```python
from build123d import *

# Parameters (mm, degrees)
F0_W            = 25
F0_H            = 50
F0_R            = 5
F1_DEPTH        = 15
F1_DEPTH_BACK   = 15
F2_COUNT        = 2
F2_ANGLE        = 90
F3_R            = 30
F4_DEPTH        = 50
F5_W            = 10
F5_H            = 64.0000030398
F6_DEPTH        = 50.0010001
F6_COPIES_COUNT = 4


# Not quite as in the source:
# - a pattern or mirror of a feature is missing from the dataset's text; its kind, count and spacing are read off the source's solid


with BuildPart() as f1:
    # F0 (on Front) → F1 (new body, two sides)
    with BuildSketch(Plane.XZ) as f1_sk:
        with Locations((-12.5, 25)):
            Rectangle(F0_W, F0_H)
        with Locations((12.5, 25)):
            Rectangle(F0_W, F0_H)
        with BuildLine():
            ThreePointArc((-25, 50), (-50, 25), (-25, 0))
            Line((-25, 0), (-25, 50))
        make_face()
        with Locations((-39.1249991953, 25)):
            Circle(F0_R, mode=Mode.SUBTRACT)
        with BuildLine():
            Line((25, 50), (25, 0))
            ThreePointArc((25, 0), (50, 25), (25, 50))
        make_face()
        with Locations((39.1249991953, 25)):
            Circle(F0_R, mode=Mode.SUBTRACT)
    extrude(amount=F1_DEPTH)
    extrude(f1_sk.sketch, amount=-F1_DEPTH_BACK)

    # F2: F1 ×2 about axis
    f2_axis = Axis((0, 0, 10.6249991804), (0, 0, 1))


with BuildPart() as f1_1:
    add(f1.part)
    for i in range(1, F2_COUNT):
        add(f1.part.rotate(f2_axis, i * F2_ANGLE / (F2_COUNT - 1)))

    # F3 (on face) → F4 (join, through all)
    with BuildSketch(Plane.XY.offset(50)):
        Circle(F3_R)
    extrude(amount=-F4_DEPTH)

    # F5 (on face) → F6 (cut, through all)
    with BuildSketch(Plane.XY.offset(50)):
        with Locations((0, 64.1250014305)):
            Rectangle(F5_W, F5_H)
    f6 = extrude(amount=-F6_DEPTH, mode=Mode.SUBTRACT)

    # F6_copies: F6 ×4 about axis
    f6_copies_axis = Axis((0, 0, 0), (0, 0, 1))
    for i in range(1, F6_COPIES_COUNT):
        add(f6.rotate(f6_copies_axis, i * 360 / F6_COPIES_COUNT), mode=Mode.SUBTRACT)


solid = f1_1.part
```
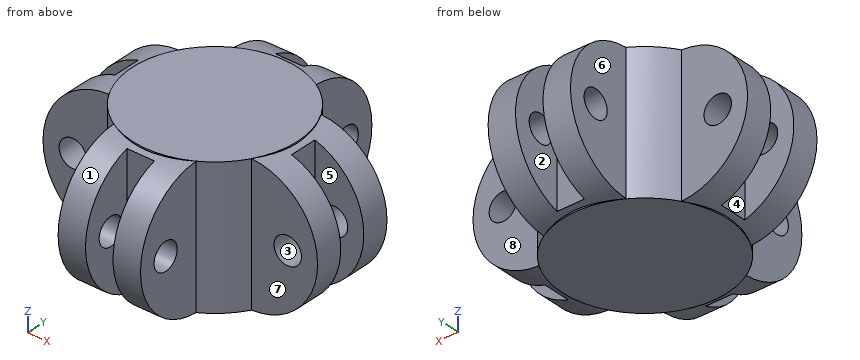
Design review of the part built by this model. Coordinates are the model's own, in mm. Face numbers are marked on the shaded views. A direction names the side the tool comes from. Round coordinates to 2 decimals unless told otherwise and drop trailing zeros. Write each loop counter-clockwise with the first axis right and the second up, starting at its lowest first coordinate (ties: lowest second). Pieces come first, ordered by that corner, then holes.
Item 1: We need section A-A on x = -13.5. Write out the cut boundary in (y, z) (3 decimals), and give its area (3 significant figures).
Item 2: We need section B-B on y = 35.5. Write out the cut boundary in (x, z), and give its area (3 significant figures).
Item 3: For the marked faces 4, 5, 6, 7 and 8, list the 3-axis set-ups (+Z, -Z, +X, -X, +Y, -Y) from which the entire face can be reached by the end or side of a thin tool; tool diameter is ignored.
Item 4: Clearance check with flat-ended pins moving along their axes: pin 1 Ø12 at (x, z) = (23.5, 41.5) entering from -Y; pin 2 Ø7 at (x, z) = (-40, 17) entering from +Y; pin 3 Ø3 at (y, z) = (-1, 28.5) entering from +X (3 decimals); pin 4 Ø6 at (x, z) = (-39.125, 25) entering from -Y. State where each tip first meets the part, or that it passes through.
Item 5: We need section D-D on y = -7. Write out the cut boundary in (x, z) (3 decimals).
Item 6: We need section C-C on z = 25. State how many separate pieces and enclosed holes the cut face has, and give its area (3 significant figures).
Item 7: The part is to be moulded in two halves that separate along Z. For the marked faces 1, 2 and 3, say which applies: +Z half, -Z half, draft (parallel to the pull), parting line (faces both ways), or undercut.
Item 8: For probe 1 along Y at (x, z) = (-12, 25) (3 decimals); probe 2 along X at (y, z) = (-34, 35); probe 3 along Y at (x, z) = (26.5, 28), list the stretches that pass through material, from the lowest coordinate up.
Returned:
1. outline: (-26.791, 0) - (26.791, 0) - (26.791, 0.064) arc R25 ccw to (26.791, 49.936) - (26.791, 50) - (-26.791, 50) - (-26.791, 49.936) arc R25 ccw to (-26.791, 0.064) - close; hole circle Ø10 at (-39.125, 25); hole circle Ø10 at (39.125, 25)
1. area: 4,310 mm2
2. outline: (-15, 2.31) - (-5, 2.31) - (-5, 21.56) - (-15, 21.56) - close; (-15, 28.44) - (-5, 28.44) - (-5, 47.69) - (-15, 47.69) - close; (5, 2.31) - (15, 2.31) - (15, 21.56) - (5, 21.56) - close; (5, 28.44) - (15, 28.44) - (15, 47.69) - (5, 47.69) - close
2. area: 770 mm2
3. face 4: +Z, -Z, -X
3. face 5: +Z, -Z, +X
3. face 6: +Z, -Z, -X, +Y
3. face 7: +Z, -Z, +X, -Y
3. face 8: +Z, -Z, +X, +Y
4. pin 1: stops at y = -24.37
4. pin 2: stops at y = 15
4. pin 3: stops at x = 32.125
4. pin 4: passes through
5. outline: (-29.172, 0) - (29.172, 0) - (29.172, 0.351) arc R25 ccw to (29.172, 49.649) - (29.172, 50) - (-29.172, 50) - (-29.172, 49.649) arc R25 ccw to (-29.172, 0.351) - close; hole circle Ø10 at (-39.125, 25); hole circle Ø10 at (39.125, 25)
6. separate pieces: 9
6. enclosed holes: 0
6. area: 3,870 mm2
7. face 1: parting line
7. face 2: draft
7. face 3: undercut
8. probe 1: y = -50 to -44.125, -34.125 to 34.125, 44.125 to 50
8. probe 2: x = -15 to -5, 5 to 15
8. probe 3: y = -15 to 15
